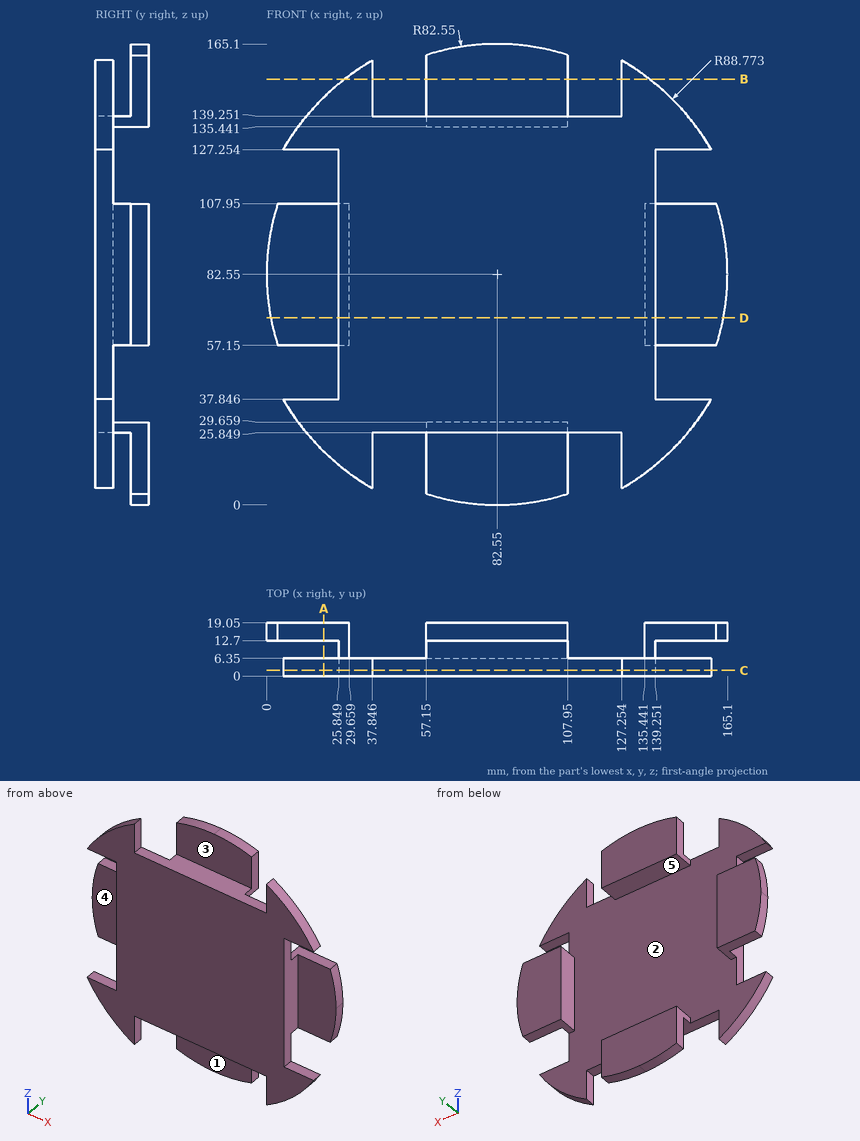
Can you work these out from the drawing? Everything is in mm from the part's minimum corner. A direction names the side the tool comes from. Coordinates: 2 decimals unless noted, no trailing zeros. Loops run counter-clockwise (first coordinate to the right, second up) from the corner with the lowest first, then second, coordinate; pieces in that order, holes last.
1. Imagine slicing it at C-C, the plane y = 2. Please give me the cut outline in (x, z), and give its area (3 significant figures).
2. Imagine slicing it at A-A, the plane x = 20.5. Please give me the cut outline in (y, z), and give its area (3 significant figures).
3. For the marked faces 3, 4 and 5, which set-ups out of +Z, -Z, +X, -X, +Y, -Y let a thin tool reach every point of the face, with its end or its side?
4. Imagine slicing it at D-D, the plane z = 67. Please give me the cut outline in (x, y), and give its area (3 significant figures).
5. Imagine slicing it at B-B, the plane z = 152.5. Please give me the cut outline in (x, y), and give its area (3 significant figures).
6. If we mould it in two halves opening along X, with no side actions, what happens to the marked faces 1 and 2? For each: pulls with the +X half, pulls with the -X half, needs draft (parallel to the pull), parting line crosses it, or undercut.
7. For P1, Ø4, axis at x = 82, y = 6, coming from the +Z side; P2, Ø6.5, axis at x = 65, y = 8.5, coming from the -Z side; P3, Ø6.5, axis at x = 79.5, y = 10, coming from the -Z side, each with a flat end and sliding along its axis, tell me the tip position at first contact or that it passes through.
8. I need wall thicknesses on L1, parallel to X at y = 10.25, z = 90; L2, parallel to Z at x = 27, y = 15.5. Which ranges of each line are inside material? Lowest first, please.
Taken from the geometry:
1. outline: (5.85, 37.85) arc R88.77 ccw to (37.85, 5.85) - (37.85, 25.85) - (127.25, 25.85) - (127.25, 5.85) arc R88.77 ccw to (159.25, 37.85) - (139.25, 37.85) - (139.25, 127.25) - (159.25, 127.25) arc R88.77 ccw to (127.25, 159.25) - (127.25, 139.25) - (37.85, 139.25) - (37.85, 159.25) arc R88.77 ccw to (5.85, 127.25) - (25.85, 127.25) - (25.85, 37.85) - close
1. area: 14,700 mm2
2. outline: (0, 19.06) - (6.35, 19.06) - (6.35, 37.85) - (0, 37.85) - close; (0, 127.25) - (6.35, 127.25) - (6.35, 146.04) - (0, 146.04) - close; (12.7, 57.15) - (19.05, 57.15) - (19.05, 107.95) - (12.7, 107.95) - close
2. area: 561 mm2
3. face 3: +Z, +X, -X, -Y
3. face 4: +Z, -Z, -X, -Y
3. face 5: +X, -X, +Y
4. outline: (1.48, 12.7) - (25.85, 12.7) - (25.85, 0) - (139.25, 0) - (139.25, 12.7) - (163.62, 12.7) - (163.62, 19.05) - (135.44, 19.05) - (135.44, 6.35) - (29.66, 6.35) - (29.66, 19.05) - (1.48, 19.05) - close
4. area: 1,130 mm2
5. outline: (27.89, 0) - (37.85, 0) - (37.85, 6.35) - (27.89, 6.35) - close; (57.15, 12.7) - (107.95, 12.7) - (107.95, 19.05) - (57.15, 19.05) - close; (127.25, 0) - (137.21, 0) - (137.21, 6.35) - (127.25, 6.35) - close
5. area: 449 mm2
6. face 1: needs draft
6. face 2: undercut
7. P1: stops at z = 139.25
7. P2: stops at z = 25.85
7. P3: stops at z = 0.01
8. L1: x = 25.85 to 29.66, 135.44 to 139.25
8. L2: z = 57.15 to 107.95
